from build123d import *

# Parameters (mm, degrees)
BOSS_EXTRUDE1_DEPTH             = 5
CUT_EXTRUDE1_REACH              = 19.493
SKETCH2_R                       = 2
BOSS_EXTRUDE2_DEPTH             = 5
CUT_EXTRUDE4_DEPTH              = 17.5
CUT_EXTRUDE10_START             = 17.5
CUT_EXTRUDE10_DEPTH             = 16
SKETCH15_W                      = 3.25
SKETCH15_H                      = 4.2
CUT_EXTRUDE11_DEPTH             = 3.8
CHAMFER2_START                  = 1.5
CHAMFER2_DEPTH                  = 4.2
CHAMFER2_START_2                = 10.3
CHAMFER2_2_DEPTH                = 4.2
CUT_EXTRUDE7_START              = -15
CUT_EXTRUDE7_DEPTH              = 28.5
BOSS_EXTRUDE7_DEPTH             = 2.5
BOSS_EXTRUDE8_DEPTH             = 2
BOSS_EXTRUDE8_DIRECTION_2_REACH = 33.286
SKETCH17_W                      = 10
SKETCH17_H                      = 9
BOSS_EXTRUDE10_DEPTH            = 2
CUT_EXTRUDE12_START             = 18
CUT_EXTRUDE12_DEPTH             = 2
CUT_EXTRUDE13_START             = 2
CUT_EXTRUDE13_DEPTH             = 2
CUT_EXTRUDE14_START             = 0.5
CUT_EXTRUDE14_DEPTH             = 0.5
FILLET8_SIZE                    = 2
FILLET8_SIZE_2                  = 1
FILLET6_SIZE                    = 1
FILLET6_SIZE_2                  = 2
CHAMFER3_SIZE                   = 2


with BuildPart() as part:
    # Sketch1 → Boss-Extrude1 (new, symmetric)
    with BuildSketch(Plane(origin=(0, 0, 0), x_dir=(0, 0, -1), z_dir=(1, 0, 0))):
        with BuildLine():
            Line((-5, -15), (-5, -7.5))
            add(Edge.make_bspline(
                [(-5, -7.5), (-4.98696359, -3.758210307), (-9, -2)],
                knots=[0, 0, 0, 1, 1, 1], degree=2))
            Line((-9, -2), (-9, 16))
            Line((-9, 16), (0, 16))
            Line((0, 16), (0, 0))
            Line((0, 0), (0, -15))
            Line((0, -15), (-5, -15))
        make_face()
    extrude(amount=BOSS_EXTRUDE1_DEPTH, both=True)

    # Sketch2 → Cut-Extrude1 (cut, up to next)
    with BuildSketch(Plane.XY.offset(5), mode=Mode.PRIVATE) as cut_extrude1_sk1:
        with Locations((0, -11.25)):
            Circle(SKETCH2_R)
    cut_extrude1_tool1 = extrude(cut_extrude1_sk1.sketch, amount=-CUT_EXTRUDE1_REACH, mode=Mode.PRIVATE) & part.part
    add(cut_extrude1_tool1.solids().sort_by_distance((0, -11.25, 5))[0], mode=Mode.SUBTRACT)

    # Sketch5 → Boss-Extrude2 (add, symmetric)
    with BuildSketch(Plane(origin=(0, 0, 0), x_dir=(0, 0, -1), z_dir=(1, 0, 0))):
        with BuildLine():
            Line((1.5, 13.5), (0, 13.5))
            Line((0, 13.5), (0, 16))
            add(Edge.make_bspline(
                [(1.5, 13.5), (1.5, 15.23543045), (1.140641964, 16), (0, 16)],
                knots=[0, 0, 0, 0, 1, 1, 1, 1], degree=3))
        make_face()
    extrude(amount=BOSS_EXTRUDE2_DEPTH, both=True)

    # Sketch6 → Cut-Extrude4 (cut)
    with BuildSketch(Plane(origin=(0, 16, 0), x_dir=(1, 0, 0), z_dir=(0, 1, 0))):
        with BuildLine():
            ThreePointArc((2.049390153, -2.9), (0, -1.9), (-2.049390153, -2.9))
            Line((-2.049390153, -2.9), (2.049390153, -2.9))
        make_face()
        with BuildLine():
            Line((2.049390153, -2.9), (-2.049390153, -2.9))
            ThreePointArc((-2.049390153, -2.9), (-0.846045389, -6.958496939), (2.6, -4.5))
            ThreePointArc((2.6, -4.5), (2.458496939, -3.653954611), (2.049390153, -2.9))
        make_face()
    extrude(amount=-CUT_EXTRUDE4_DEPTH, mode=Mode.SUBTRACT)

    # Sketch13 → Cut-Extrude10 (cut)
    with BuildSketch(Plane(origin=(0, 0, 0), x_dir=(1, 0, 0), z_dir=(0, 1, 0)).offset(CUT_EXTRUDE10_START)):
        with BuildLine():
            ThreePointArc((1.75, -6.422888452), (0, -7.1), (-1.75, -6.422888452))
            add(Edge.make_bspline(
                [(-1.75, -6.422888452), (-1.75, -7.3), (-2.5, -6.8), (-2.5, -9)],
                knots=[0, 0, 0, 0, 1, 1, 1, 1], degree=3))
            Line((-2.5, -9), (2.5, -9))
            add(Edge.make_bspline(
                [(1.75, -6.422888452), (1.75, -7.3), (2.5, -6.8), (2.5, -9)],
                knots=[0, 0, 0, 0, 1, 1, 1, 1], degree=3))
        make_face()
    extrude(amount=-CUT_EXTRUDE10_DEPTH, mode=Mode.SUBTRACT)

    # Sketch15 → Cut-Extrude11 (cut)
    with BuildSketch(Plane.XY.offset(9)):
        with Locations((-3.375, 3.6)):
            Rectangle(SKETCH15_W, SKETCH15_H)
        with Locations((-3.375, 12.4)):
            Rectangle(SKETCH15_W, SKETCH15_H)
    extrude(amount=-CUT_EXTRUDE11_DEPTH, mode=Mode.SUBTRACT)

    # Chamfer2: read off the stored shape, not the designer's step
    # Chamfer2 outline → Chamfer2 (cut)
    with BuildSketch(Plane(origin=(0, 0, 0), x_dir=(1, 0, 0), z_dir=(0, 1, 0)).offset(CHAMFER2_START)):
        with BuildLine():
            ThreePointArc((-2.503996805, -5.2), (-2.574603342, -4.137484302), (-2.213344965, -3.13577712))
            Line((-2.213344965, -3.13577712), (-4.130598027, -5.2))
            Line((-4.130598027, -5.2), (-2.503996805, -5.2))
        make_face()
    extrude(amount=CHAMFER2_DEPTH, mode=Mode.SUBTRACT)

    # Chamfer2 2 outline → Chamfer2 2 (cut)
    with BuildSketch(Plane(origin=(0, 0, 0), x_dir=(1, 0, 0), z_dir=(0, 1, 0)).offset(CHAMFER2_START_2)):
        with BuildLine():
            ThreePointArc((-2.503996805, -5.2), (-2.574603342, -4.137484302), (-2.213344965, -3.13577712))
            Line((-2.213344965, -3.13577712), (-4.130598027, -5.2))
            Line((-4.130598027, -5.2), (-2.503996805, -5.2))
        make_face()
    extrude(amount=CHAMFER2_2_DEPTH, mode=Mode.SUBTRACT)

    # Sketch9 → Cut-Extrude7 (cut)
    with BuildSketch(Plane(origin=(0, 0, 0), x_dir=(1, 0, 0), z_dir=(0, 1, 0)).offset(CUT_EXTRUDE7_START)):
        with BuildLine():
            Line((5, 0), (-5, 0))
            ThreePointArc((-5, 0), (0, -0.138996222), (5, 0))
        make_face()
    extrude(amount=CUT_EXTRUDE7_DEPTH, mode=Mode.SUBTRACT)

    # Sketch12 → Boss-Extrude7 (add)
    with BuildSketch(Plane.XZ.offset(-13.5)):
        with BuildLine():
            Line((5, 0), (-5, 0))
            Line((-5, 0), (-5, -0.75))
            ThreePointArc((-5, -0.75), (-7.356122713, -1.757737527), (-9.249008864, -3.485114493))
            Line((-9.249008864, -3.485114493), (-7.446859958, -3.218783834))
            Line((-7.446859958, -3.218783834), (-6.860693731, -7.185127133))
            Line((-6.860693731, -7.185127133), (5, -7.185127133))
            Line((5, -7.185127133), (5, 0))
        make_face()
    extrude(amount=-BOSS_EXTRUDE7_DEPTH)

    # Sketch12<4> → Boss-Extrude8 (add)
    with BuildSketch(Plane.XZ.offset(-13.5)):
        with BuildLine():
            Line((-9.249008864, -3.485114493), (-7.446859958, -3.218783834))
            Line((-7.446859958, -3.218783834), (-6.860693731, -7.185127133))
            ThreePointArc((-6.860693731, -7.185127133), (-8.565464188, -5.664715496), (-9.249008864, -3.485114493))
        make_face()
    extrude(amount=BOSS_EXTRUDE8_DEPTH)

    # Boss-Extrude8 direction 2: up to this face of the body (flat: up to its plane)
    boss_extrude8_direction_2_end = Plane(part.part.faces().sort_by_distance((-0.643733598, 16, -0.592776419))[0])
    # Sketch12<4> → Boss-Extrude8 direction 2 (add, up to the picked face)
    with BuildSketch(Plane.XZ.offset(-13.5), mode=Mode.PRIVATE) as boss_extrude8_direction_2_sk1:
        with BuildLine():
            Line((-9.249008864, -3.485114493), (-7.446859958, -3.218783834))
            Line((-7.446859958, -3.218783834), (-6.860693731, -7.185127133))
            ThreePointArc((-6.860693731, -7.185127133), (-8.565464188, -5.664715496), (-9.249008864, -3.485114493))
        make_face()
    boss_extrude8_direction_2_tool1 = split(extrude(boss_extrude8_direction_2_sk1.sketch, amount=-BOSS_EXTRUDE8_DIRECTION_2_REACH, mode=Mode.PRIVATE), bisect_by=boss_extrude8_direction_2_end, keep=Keep.BOTH, mode=Mode.PRIVATE)
    add(boss_extrude8_direction_2_tool1.solids().sort_by(Axis((-7.987517, 13.5, -4.907532), (0, 1, 0)))[0])

    # Sketch17 → Boss-Extrude10 (add)
    with BuildSketch(Plane(origin=(0, 16, 0), x_dir=(1, 0, 0), z_dir=(0, 1, 0))):
        with Locations((0, -4.5)):
            Rectangle(SKETCH17_W, SKETCH17_H)
    extrude(amount=BOSS_EXTRUDE10_DEPTH)

    # Sketch13<3> → Cut-Extrude12 (cut)
    with BuildSketch(Plane(origin=(0, 0, 0), x_dir=(1, 0, 0), z_dir=(0, 1, 0)).offset(CUT_EXTRUDE12_START)):
        with BuildLine():
            Line((-2.5, -9), (2.5, -9))
            add(Edge.make_bspline(
                [(1.75, -6.422888452), (1.75, -7.3), (2.5, -6.8), (2.5, -9)],
                knots=[0, 0, 0, 0, 1, 1, 1, 1], degree=3))
            ThreePointArc((1.75, -6.422888452), (0, -7.1), (-1.75, -6.422888452))
            add(Edge.make_bspline(
                [(-1.75, -6.422888452), (-1.75, -7.3), (-2.5, -6.8), (-2.5, -9)],
                knots=[0, 0, 0, 0, 1, 1, 1, 1], degree=3))
        make_face()
    extrude(amount=-CUT_EXTRUDE12_DEPTH, mode=Mode.SUBTRACT)

    # Sketch6<4> → Cut-Extrude13 (cut)
    with BuildSketch(Plane(origin=(0, 16, 0), x_dir=(1, 0, 0), z_dir=(0, 1, 0)).offset(CUT_EXTRUDE13_START)):
        with BuildLine():
            Line((2.049390153, -2.9), (-2.049390153, -2.9))
            ThreePointArc((-2.049390153, -2.9), (-0.846045389, -6.958496939), (2.6, -4.5))
            ThreePointArc((2.6, -4.5), (2.458496939, -3.653954611), (2.049390153, -2.9))
        make_face()
    extrude(amount=-CUT_EXTRUDE13_DEPTH, mode=Mode.SUBTRACT)

    # Sketch6<5> → Cut-Extrude14 (cut)
    with BuildSketch(Plane(origin=(0, 16, 0), x_dir=(1, 0, 0), z_dir=(0, 1, 0)).offset(CUT_EXTRUDE14_START)):
        with BuildLine():
            ThreePointArc((2.049390153, -2.9), (0, -1.9), (-2.049390153, -2.9))
            Line((-2.049390153, -2.9), (2.049390153, -2.9))
        make_face()
        with BuildLine():
            Line((2.049390153, -2.9), (-2.049390153, -2.9))
            ThreePointArc((-2.049390153, -2.9), (-0.846045389, -6.958496939), (2.6, -4.5))
            ThreePointArc((2.6, -4.5), (2.458496939, -3.653954611), (2.049390153, -2.9))
        make_face()
    extrude(amount=-CUT_EXTRUDE14_DEPTH, mode=Mode.SUBTRACT)

    # Fillet8
    # a fillet whose section is not a circle: 2, 1 mm, written as the material it takes off along each edge
    with BuildSketch(Plane(origin=(5, 23, 9), x_dir=(-1, 0, 0), z_dir=(0, -1, 0))) as fillet8_piece_1:
        with BuildLine():
            Bezier((FILLET8_SIZE, 0), (0, 0), (0, FILLET8_SIZE_2), weights=[1, 0.707106781, 1])
            Line((0, FILLET8_SIZE_2), (0, 0))
            Line((0, 0), (FILLET8_SIZE, 0))
        make_face()
    extrude(amount=30, mode=Mode.SUBTRACT)

    # Fillet6
    # a fillet whose section is not a circle: 2, 1 mm, written as the material it takes off along each edge
    with BuildSketch(Plane(origin=(-5, -7, 9), x_dir=(0, 0, -1), z_dir=(0, 1, 0)), Plane(origin=(-5, 9.5, 9), x_dir=(0, 0, -1), z_dir=(0, 1, 0))) as fillet6_piece_1:
        with BuildLine():
            Bezier((FILLET6_SIZE, 0), (0, 0), (0, -FILLET6_SIZE_2), weights=[1, 0.707106781, 1])
            Line((0, -FILLET6_SIZE_2), (0, 0))
            Line((0, 0), (FILLET6_SIZE, 0))
        make_face()
    extrude(amount=13.5, mode=Mode.SUBTRACT)
    with BuildSketch(Plane(origin=(-5, 0.7, 9), x_dir=(0, 0, -1), z_dir=(0, 1, 0))) as fillet6_piece_2:
        with BuildLine():
            Bezier((FILLET6_SIZE, 0), (0, 0), (0, -FILLET6_SIZE_2), weights=[1, 0.707106781, 1])
            Line((0, -FILLET6_SIZE_2), (0, 0))
            Line((0, 0), (FILLET6_SIZE, 0))
        make_face()
    extrude(amount=14.6, mode=Mode.SUBTRACT)

    # Chamfer3
    chamfer3_edges = [part.edges().sort_by_distance(p)[0] for p in [
        (0, 16, 0),
    ]]
    chamfer(chamfer3_edges, length=CHAMFER3_SIZE - 0.0001)  # a hair under: the kernel refuses the full size


solid = part.part
Design review of the part built by this model. Coordinates are the model's own, in mm. A direction names the side the tool comes from. Coordinates: 2 decimals unless noted, no trailing zeros. Order: outer loops, then holes, each group sorted by start corner. A loop starts at its lowest first (then second) coordinate and runs counter-clockwise, first axis right, second up. Notation, with made-up numbers: M 32,61 L 37,61 A24 ccw 37,98 Z; hole C -13,43 d2. An arc over 180 degrees is marked long. Use a Markdown table: item, result.
(1) Add section A-A (y = -11.25). Give the boundary of the cut face in (x, z), then the cut area to 3 significant figures.
Worked answers:
| item | result |
|---|---|
| outline | M -5,0 A90 cw -2,0.12 L -2,5 L -5,5 Z; M 2,0.12 A90 cw 5,0 L 5,5 L 2,5 Z |
| area | 29.6 mm2 |
(2) For P1, Ø7, axis at y = 7, z = 2.5, coming from the -X side; P2, Ø2, axis at x = -1.5, z = -4, coming from the -Y side; P3, Ø6, axis at x = 2, y = -10, coming from the +Z side, all flat-tipped, find the tip position at first contact; note any pin that passes through.
Worked answers:
| item | result |
|---|---|
| P1 | stops at x = -5 |
| P2 | stops at y = 13.5 |
| P3 | stops at z = 5.02 |
(3) Add section D-D (z = -5.75). Give the boundary of the cut face in (x, y), then the cut area to 3 significant figures.
Worked answers:
| item | result |
|---|---|
| outline | M -8.51,11.5 L -7.07,11.5 L -7.07,13.5 L 5,13.5 L 5,16 L -8.51,16 Z |
| area | 36.6 mm2 |
(4) Add section B-B (z = 4.5). Give the boundary of the cut face in (x, y), then the cut area to 3 significant figures.
Worked answers:
| item | result |
|---|---|
| outline | M -5,-15 L 5,-15 L 5,18 L 2.6,18 L 2.6,-1.5 L -2.6,-1.5 L -2.6,1.5 L -3.48,1.5 L -3.48,5.7 L -2.6,5.7 L -2.6,10.3 L -3.48,10.3 L -3.48,14.5 L -2.6,14.5 L -2.6,18 L -5,18 Z; hole C 0,-11.25 d4 |
| area | 209 mm2 |
(5) Wall thickness on probe 1 along Y at (x, z) = (0, 2.4); probe 2 along X at (y, z) = (-11.25, 2.7); probe 3 along X at (y, z) = (13, 4.5): over which ranges is each line inside the solid? List them lowest first.
Worked answers:
| item | result |
|---|---|
| probe 1 | y = -15 to -13.25, -9.25 to -1.5, 16.5 to 18 |
| probe 2 | x = -5 to -2, 2 to 5 |
| probe 3 | x = -5 to -3.48, 2.6 to 5 |
(6) Draft analysis for pull direction Z (two halves, no side actions). For faces 4 (the flat face through (-8.361, 12.514, -3.354)), 5 (the cylindrical face through (-0.07, -0.95, 0.14)), 6 (the flat face through (0, -1.5, 4)), 7 (the flat face through (-2, 1.5, 7)), state which applies: released by +Z, released by -Z, zero draft, split by the parting line, or undercut.
Worked answers:
| item | result |
|---|---|
| face 4 | released by +Z |
| face 5 | released by -Z |
| face 6 | undercut |
| face 7 | zero draft |
(7) For faces 1 (the flat face through (-5, 1, 4)), 2 (the flat face through (-4.6, 3.6, 5.2)), 3 (the flat face through (-3.2, 3.6, 4.2)), list the 3-axis set-ups (+Z, -Z, +X, -X, +Y, -Y) from which the entire face can be reached by the end or side of a thin tool; tool diameter is ignored.
Worked answers:
| item | result |
|---|---|
| face 1 | +Z, -X, +Y, -Y |
| face 2 | +Z, -X |
| face 3 | +Z |
(8) Add section C-C (x = -5.5). Give the boundary of the cut face in (y, z), then the cut area to 3 significant figures.
Worked answers:
| item | result |
|---|---|
| outline | M 13.5,-7.19 L 16,-7.19 L 16,-2 L 17.11,-0.89 L 13.5,-0.89 Z |
| area | 16.4 mm2 |
